Autodesk Inventor part; units mm, degrees
ref_plane "YZ Plane" through (0, 0, 0) normal (1, 0, 0) x (0, 1, 0)
ref_plane "XZ Plane" through (0, 0, 0) normal (0, 1, 0) x (-1, 0, 0)
ref_plane "XY Plane" through (0, 0, 0) normal (0, 0, 1) x (1, 0, 0)
sketch "Sketch1" plane through (0, 0, 0) normal (1, 0, 0) x (0, 1, 0)
  circle A0 centre (8.9201, -5.15) radius 5.15
  circle A1 centre (8.9201, 5.15) radius 5.15
  circle A2 centre (0, 10.3) radius 5.15
  circle A3 centre (-8.9201, 5.15) radius 5.15
  circle A4 centre (-8.9201, -5.15) radius 5.15
  circle A5 centre (0, -10.3) radius 5.15
  line L0 (-27.5, 7.5) -> (-16.5, 7.5)
  line L1 (-16.5, 7.5) -> (-16.5, -7.5)
  line L2 (-16.5, -7.5) -> (-27.5, -7.5)
  line L3 (-27.5, -7.5) -> (-27.5, 7.5)
  line L4 (-27.5, 7.5) -> (-16.5, -7.5) construction
  line L5 (-16.5, 7.5) -> (-27.5, -7.5) construction
  line L6 (14.7452, -10.5394) -> (20.2452, -20.0657)
  line L7 (1.7548, -18.0394) -> (14.7452, -10.5394)
  line L8 (7.2548, -27.5657) -> (1.7548, -18.0394)
  line L9 (20.2452, -20.0657) -> (7.2548, -27.5657)
  line L10 (1.7548, 18.0394) -> (7.2548, 27.5657)
  line L11 (14.7452, 10.5394) -> (1.7548, 18.0394)
  line L12 (20.2452, 20.0657) -> (14.7452, 10.5394)
  line L13 (7.2548, 27.5657) -> (20.2452, 20.0657)
  circle A6 centre (-22, 25) radius 3.25
  circle A7 centre (-22, -25) radius 3.25
  arc A8 (-22, 31) -> (-28, 25) centre (-22, 25) ccw
  arc A9 (-28, -25) -> (-22, -31) centre (-22, -25) ccw
  line L14 (-28, 25) -> (-28, -25)
  line L15 (-22, 31) -> (10, 31)
  line L16 (10, -31) -> (-22, -31)
  line L17 (10, -31) -> (24, -22.9171)
  line L18 (24, -22.9171) -> (24, 22.9171)
  line L19 (24, 22.9171) -> (10, 31)
  point P0 (0, 0)
  point P1 (-22, 0)
  point P2 (-4.46, -7.725)
  point P3 (-8.9201, 0)
  point P4 (-4.46, 7.725)
  point P5 (4.46, 7.725)
  point P6 (8.9201, 0)
  point P7 (4.46, -7.725)
  dimension "d0" = 10.3
  dimension "d3" = 360
  dimension "d5" = 15
  dimension "d6" = 11
  dimension "d7" = 22
  dimension "d10" = 360
  dimension "d12" = 25
  dimension "d13" = 50
  dimension "d14" = 6.5
  dimension "d15" = 12
  dimension "d29" = 10
  dimension "d31" = 24
extrude "Layer1_Magnets_16" add sketch "Sketch1" along normal blind 1.6 contours A0 A5 A4 A3 A2 A1 | L15 L19 L18 L17 L16 A9 L14 A8
sketch "Sketch2" plane through (1.6, 0, 0) normal (1, 0, 0) x (0, 0, -1)
  arc A0 (-31, -22) -> (-25, -28) centre (-25, -22) ccw
  line L0 (-25, -28) -> (25, -28)
  arc A1 (25, -28) -> (31, -22) centre (25, -22) ccw
  line L1 (31, -22) -> (31, 10)
  line L2 (-31, 10) -> (-31, -22)
  arc A2 (7.725, -4.46) -> (7.725, 4.46) centre (10.3, 0) ccw
  arc A3 (0, -8.9201) -> (7.725, -4.46) centre (5.15, -8.9201) ccw
  arc A4 (-7.725, -4.46) -> (0, -8.9201) centre (-5.15, -8.9201) ccw
  arc A5 (-7.725, 4.46) -> (-7.725, -4.46) centre (-10.3, 0) ccw
  arc A6 (0, 8.9201) -> (-7.725, 4.46) centre (-5.15, 8.9201) ccw
  arc A7 (7.725, 4.46) -> (0, 8.9201) centre (5.15, 8.9201) ccw
  circle A8 centre (25, -22) radius 3.25
  circle A9 centre (-25, -22) radius 3.25
  line L3 (-18.0394, 1.7548) -> (-27.5657, 7.2548)
  line L4 (-27.5657, 7.2548) -> (-20.0657, 20.2452)
  line L5 (-20.0657, 20.2452) -> (-10.5394, 14.7452)
  line L6 (-10.5394, 14.7452) -> (-18.0394, 1.7548)
  line L7 (10.5394, 14.7452) -> (20.0657, 20.2452)
  line L8 (20.0657, 20.2452) -> (27.5657, 7.2548)
  line L9 (27.5657, 7.2548) -> (18.0394, 1.7548)
  line L10 (18.0394, 1.7548) -> (10.5394, 14.7452)
  line L11 (-7.5, -27.5) -> (-7.5, -16.5)
  line L12 (-7.5, -16.5) -> (7.5, -16.5)
  line L13 (7.5, -16.5) -> (7.5, -27.5)
  line L14 (7.5, -27.5) -> (-7.5, -27.5)
  arc A10 (0, 8.9201) -> (7.725, 4.46) centre (5.15, 8.9201) ccw
  arc A11 (-7.725, 4.46) -> (0, 8.9201) centre (-5.15, 8.9201) ccw
  arc A12 (-7.725, -4.46) -> (-7.725, 4.46) centre (-10.3, 0) ccw
  arc A13 (0, -8.9201) -> (-7.725, -4.46) centre (-5.15, -8.9201) ccw
  arc A14 (7.725, -4.46) -> (0, -8.9201) centre (5.15, -8.9201) ccw
  arc A15 (7.725, 4.46) -> (7.725, -4.46) centre (10.3, 0) ccw
  line L15 (31, 10) -> (22.9171, 24)
  line L16 (22.9171, 24) -> (-22.9171, 24)
  line L17 (-22.9171, 24) -> (-31, 10)
  point P0 (0, 0)
  point P1 (-7.725, 4.46)
  point P2 (-7.725, 4.46)
  point P3 (-7.725, 4.46)
  point P4 (-7.725, -4.46)
  point P5 (-7.725, -4.46)
  point P6 (-7.725, -4.46)
  point P7 (-7.725, -4.46)
  point P8 (0, -8.9201)
  point P9 (0, -8.9201)
  point P10 (0, -8.9201)
  point P11 (7.725, 4.46)
  point P12 (7.725, 4.46)
  point P13 (0, 8.9201)
  point P14 (0, 8.9201)
extrude "Layer2_Coupler_80" add sketch "Sketch2" along normal blind 6.4 contours L2 L17 L16 L15 L1 A1 L0 A0 | A15 A2 | A3 A14 | A14 A13 A12 A11 A10 A15 | A10 A7 | A4 A13 | A11 A6 | A5 A12
sketch "Sketch3" plane through (8, 0, 0) normal (1, 0, 0) x (0, 0, -1)
  circle A0 centre (25, -22) radius 3.25
  circle A1 centre (-25, -22) radius 3.25
  line L0 (-18.0394, 1.7548) -> (-27.5657, 7.2548)
  line L1 (-27.5657, 7.2548) -> (-20.0657, 20.2452)
  line L2 (-20.0657, 20.2452) -> (-10.5394, 14.7452)
  line L3 (-10.5394, 14.7452) -> (-18.0394, 1.7548)
  line L4 (10.5394, 14.7452) -> (20.0657, 20.2452)
  line L5 (20.0657, 20.2452) -> (27.5657, 7.2548)
  line L6 (27.5657, 7.2548) -> (18.0394, 1.7548)
  line L7 (18.0394, 1.7548) -> (10.5394, 14.7452)
  line L8 (-7.5, -27.5) -> (-7.5, -16.5)
  line L9 (-7.5, -16.5) -> (7.5, -16.5)
  line L10 (7.5, -16.5) -> (7.5, -27.5)
  line L11 (7.5, -27.5) -> (-7.5, -27.5)
  line L12 (-25, -28) -> (25, -28)
  arc A2 (25, -28) -> (31, -22) centre (25, -22) ccw
  line L13 (31, -22) -> (31, 10)
  line L14 (-31, 10) -> (-31, -22)
  arc A3 (-31, -22) -> (-25, -28) centre (-25, -22) ccw
  line L15 (22.9171, 24) -> (-22.9171, 24)
  line L16 (-22.9171, 24) -> (-31, 10)
  line L17 (31, 10) -> (22.9171, 24)
  point P0 (0, 0)
extrude "Layer3_Cover_90" add sketch "Sketch3" along normal blind 1 contours L0 L1 L2 L3 | L4 L5 L6 L7 | L8 L9 L10 L11 | A3 L14 L16 L15 L17 L13 A2 L12
chamfer "CouplerL" distance 7.5 angle 45 6 edges at (8, -22, 7.5) (8, -22, -7.5) (8, 4.5048, -22.8026) (8, 17.4952, -15.3026) (8, 17.4952, 15.3026) (8, 4.5048, 22.8026)
fillet "EdgeRadius" radius 6 4 edges at (4.5, 10, -31) (4.5, 10, 31) (4.5, 24, 22.9171) (4.5, 24, -22.9171)
equation "\"d13\" = 2 * d12"
properties part number "Tool_Template" material "ABS Plastic"
Check sheet for the modelled part. Datum: model origin and axes. Units: mm. A direction names the side the tool comes from. Round coordinates to 2 decimals unless told otherwise and drop trailing zeros. Loops run counter-clockwise (first coordinate to the right, second up) from the corner with the lowest first, then second, coordinate; pieces in that order, holes last.
1. Sectioned sample at B-B on x = 6.5. Record the boundary of the cut face in (y, z).
2. Sectioned sample at C-C on z = -13. Record the boundary of the cut face in (x, y).
3. Sectioned sample at D-D on y = 6. Record the boundary of the cut face in (x, z), and give its area (3 significant figures).
4. Sectioned sample at A-A on y = 0. Record the boundary of the cut face in (x, z), and give its area (3 significant figures).
5. Scan lines: probe 1 along Z at (x, y) = (2, -22); probe 2 along Z at (x, y) = (7.75, 11); probe 3 along Y at (x, z) = (2.5, -3). Record each from-to range of solid material in increasing order.
6. Set-up check for faces 1 (the flat face through (4, -7, 31)), 2 (the flat face through (4, -22, 4)): record each of +Z, -Z, +X, -X, +Y, -Y from which the full face is reachable in a straight line by a thin tool's end or side.
7. Gauge pin test, flat ends, axial feed: pin 1 Ø5 at (y, z) = (11, -6.5) entering from -X; pin 2 Ø4 at (y, z) = (-22, 25) entering from +X; pin 3 Ø3 at (y, z) = (11.5, -20.5) entering from -X; pin 4 Ø3 at (y, z) = (11, 19) entering from -X. Record the tip position at first contact, or that the pin passes through.
8. Mould release check, pull along Z, two halves, no side actions. Record for faces 3 (the flat face through (1.6, 0, 10)), 4 (the flat face through (4, 24, 0)), 5 (the cylindrical face through (4.437, -26.196, -29.289)): released by +Z, released by -Z, zero draft, split by the parting line, or undercut.
Recorded:
1. outline: (-28, -25) arc R6 ccw to (-22, -31) - (8.39, -31) arc R6 ccw to (11.39, -30.2) - (21, -24.65) arc R6 ccw to (24, -19.45) - (24, 19.45) arc R6 ccw to (21, 24.65) - (11.39, 30.2) arc R6 ccw to (8.39, 31) - (-22, 31) arc R6 ccw to (-28, 25) - close; hole (-27.5, -1.5) - (-16.5, -1.5) - (-16.5, 1.5) - (-27.5, 1.5) - close; hole circle Ø6.5 at (-22, -25); hole circle Ø6.5 at (-22, 25); hole (6.95, -15.04) - (12.45, -24.57) - (15.05, -23.07) - (9.55, -13.54) - close; hole (6.95, 15.04) - (9.55, 13.54) - (15.05, 23.07) - (12.45, 24.57) - close
2. outline: (0, -28) - (9, -28) - (9, 24) - (0, 24) - (0, 16.17) - (0.5, 16.17) - (5.42, 10.48) - (0, 10.48) - (0, 4.39) - (1.6, 4.39) - (1.6, -4.39) - (0, -4.39) - close
3. outline: (0, -31) - (9, -31) - (9, 31) - (0, 31) - (0, 25.39) - (0.5, 25.39) - (5.4, 15.59) - (0, 15.59) - (0, 9.39) - (1.6, 9.39) - (1.6, 0.91) - (0, 0.91) - (0, -0.91) - (1.6, -0.91) - (1.6, -9.39) - (0, -9.39) - (0, -15.59) - (5.4, -15.59) - (0.5, -25.39) - (0, -25.39) - close
3. area: 473 mm2
4. outline: (0, -31) - (9, -31) - (9, 31) - (0, 31) - (0, 15.45) - (1.6, 15.45) - (1.6, 5.15) - (0, 5.15) - (0, -5.15) - (1.6, -5.15) - (1.6, -15.45) - (0, -15.45) - close
4. area: 525 mm2
5. probe 1: z = -31 to -28.25, -21.75 to -6, 6 to 21.75, 28.25 to 31
5. probe 2: z = -30.4 to -19.55, -18.55 to 18.55, 19.55 to 30.4
5. probe 3: y = -28 to -27.5, -16.5 to 24
6. face 1: +Z, +X, -X, +Y, -Y
6. face 2: -X
7. pin 1: stops at x = 1.6
7. pin 2: passes through
7. pin 3: stops at x = 6.21
7. pin 4: stops at x = 6.47
8. face 3: undercut
8. face 4: zero draft
8. face 5: released by -Z
